Here's how the part is built. I have some questions about the finished solid (model axes, mm). Face numbers are marked on the shaded views. A direction names the side the tool comes from. Give positions to 0.01 mm unless a question says otherwise; leave off trailing zeros. Loops run counter-clockwise (first coordinate to the right, second up) from the corner with the lowest first, then second, coordinate; pieces in that order, holes last. Notation, with made-up numbers: (71, 17.5) - (90, 17.5) arc R12 ccw to (90, 23.5) - close; hole circle Ø3 at (43.25, -28). An arc over 180 degrees is marked (long way). Use a Markdown table: item, result.
from build123d import *

# Parameters (mm, degrees)
SKETCH_1_R          = 1.25
EXTRUDE_1_DEPTH     = 6
SKETCH_2_R          = 2.5
EXTRUDE_2_DEPTH     = 1.5
CUT_EXTRUDE_1_DEPTH = 0.5


with BuildPart() as part:
    # 草图1 → 凸台-拉伸1 (new body)
    with BuildSketch(Plane.XY):
        Circle(SKETCH_1_R)
    extrude(amount=EXTRUDE_1_DEPTH)

    # 草图2 → 凸台-拉伸2 (add)
    with BuildSketch(Plane(origin=(0, 0, 0), x_dir=(-1, 0, 0), z_dir=(0, 0, -1))):
        Circle(SKETCH_2_R)
    extrude(amount=EXTRUDE_2_DEPTH)

    # 草图3 → 切除-拉伸1 (cut)
    with BuildSketch(Plane(origin=(0, 0, -1.5), x_dir=(-1, 0, 0), z_dir=(0, 0, -1))):
        Polygon((0.18, 1.25), (0.18, 0.18), (1.25, 0.18), (1.25, -0.18), (0.18, -0.18), (0.18, -1.25), (-0.18, -1.25), (-0.18, -0.18), (-1.25, -0.18), (-1.25, 0.18), (-0.18, 0.18), (-0.18, 1.25), align=None)
    extrude(amount=-CUT_EXTRUDE_1_DEPTH, mode=Mode.SUBTRACT)


solid = part.part
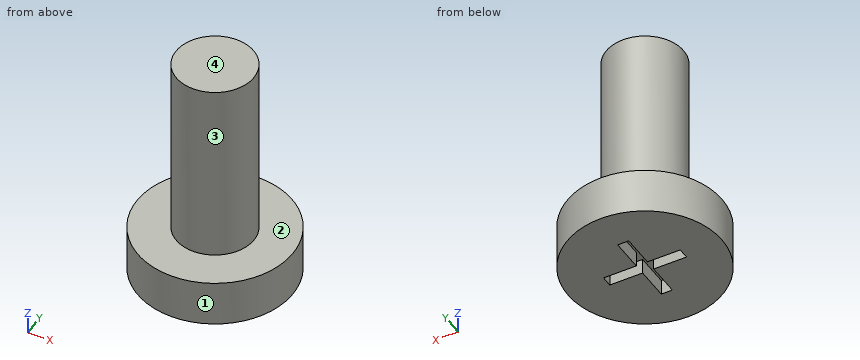
(1) If I drill on line 1 (Z direction, x = 1.2, y = 0.45); line 2 (X direction, y = -0.05, z = 1.25); line 3 (Y direction, x = -1.05, z = 5.5), over which ranges is the centre line in solid material (lowest first)?
A:
| item | result |
|---|---|
| line 1 | -1.5 to 0 |
| line 2 | -1.25 to 1.25 |
| line 3 | -0.68 to 0.68 |
(2) Will these pins go through, and if not, where does the flat tip stop? pin 1 (0.6 mm diameter, centred on x = -0.5, z = -1, fed in from -Y); pin 2 (1 mm diameter, centred on x = -1.5, z = 0, fed in from +Y); pin 3 (0.6 mm diameter, centred on y = -0.5, z = -1, fed in from +X).
A:
| item | result |
|---|---|
| pin 1 | y = -2.49 |
| pin 2 | y = 2.29 |
| pin 3 | x = 2.49 |
(3) Suppose I cut it at D-D on y = -1.5. Write out the boundary of the cut face in (x, z).
A:
| item | result |
|---|---|
| outline | (-2, -1.5) - (2, -1.5) - (2, 0) - (-2, 0) - close |
(4) Suppose I cut it at A-A on x = 0. Write out the boundary of the cut face in (y, z).
A:
| item | result |
|---|---|
| outline | (-2.5, -1.5) - (-1.25, -1.5) - (-1.25, -1) - (1.25, -1) - (1.25, -1.5) - (2.5, -1.5) - (2.5, 0) - (1.25, 0) - (1.25, 6) - (-1.25, 6) - (-1.25, 0) - (-2.5, 0) - close |
(5) We'd pull the mould along Y, two halves only. Please class the marked faces 3 and 4: pulls with the +Y half, pulls with the -Y half, needs draft (parallel to the pull), parting line crosses it, or undercut.
A:
| item | result |
|---|---|
| face 3 | parting line crosses it |
| face 4 | needs draft |
(6) On a 3-axis mill with a long thin cutter (end or side, diameter ignored), from which of +Z, -Z, +X, -X, +Y, -Y can I reach the whole of each face in a straight line? I mean the marked faces 1 and 2. Say none if no direction works.
A:
| item | result |
|---|---|
| face 1 | +Z, -Z |
| face 2 | +Z |
(7) Suppose I cut it at C-C on z = 1. Write out the boundary of the cut face in (x, y), plus the area to 3 significant figures.
A:
| item | result |
|---|---|
| outline | circle Ø2.5 at (0, 0) |
| area | 4.91 mm2 |
